```python
from build123d import *

# Parameters (mm, degrees)
SKETCH1_W           = 54.9656
SKETCH1_H           = 29.972
BOSS_EXTRUDE1_DEPTH = 21.4122
SHELL1_T            = -2.2352
SKETCH2_R           = 1.143
CUT_EXTRUDE1_DEPTH  = 38.925806526
SKETCH3_W           = 2.2352
SKETCH3_H           = 25.5016
CUT_EXTRUDE2_DEPTH  = 15.24
SKETCH4_W           = 8.981533828
SKETCH4_H           = 2.2352
SKETCH4_W_2         = 18.352338923
CUT_EXTRUDE3_DEPTH  = 19.177
SKETCH6_W           = 0.635
SKETCH6_H           = 1.8288
BOSS_EXTRUDE2_DEPTH = 5.08


with BuildPart() as part:
    # Sketch1 → Boss-Extrude1 (new body)
    with BuildSketch(Plane.XY):
        Rectangle(SKETCH1_W, SKETCH1_H)
    extrude(amount=BOSS_EXTRUDE1_DEPTH)

    # Shell1
    shell1_openings = [part.faces().sort_by_distance(p)[0] for p in [
        (0, 0, 21.4122),
    ]]
    offset(amount=SHELL1_T, openings=shell1_openings, kind=Kind.INTERSECTION)

    # Sketch2 → Cut-Extrude1 (cut, through all)
    with BuildSketch(Plane(origin=(0, 0, 0), x_dir=(-1, 0, 0), z_dir=(0, 0, -1))):
        with Locations((1.7018, 11.176)):
            Circle(SKETCH2_R)
        with Locations((-11.7856, -11.176)):
            Circle(SKETCH2_R)
        with Locations((15.1892, -11.176)):
            Circle(SKETCH2_R)
    extrude(amount=-CUT_EXTRUDE1_DEPTH, mode=Mode.SUBTRACT)

    # Sketch3 → Cut-Extrude2 (cut)
    with BuildSketch(Plane.XY.offset(21.4122)):
        with Locations((26.3652, 0)):
            Rectangle(SKETCH3_W, SKETCH3_H)
    extrude(amount=-CUT_EXTRUDE2_DEPTH, mode=Mode.SUBTRACT)

    # Sketch4 → Cut-Extrude3 (cut)
    with BuildSketch(Plane.XY.offset(21.4122)):
        with Locations((10.870255505, -13.8684)):
            Rectangle(SKETCH4_W, SKETCH4_H)
        with Locations((4.107846369, 13.8684)):
            Rectangle(SKETCH4_W_2, SKETCH4_H)
    extrude(amount=-CUT_EXTRUDE3_DEPTH, mode=Mode.SUBTRACT)

    # Sketch6 → Boss-Extrude2 (add)
    with BuildSketch(Plane.ZY.offset(27.4828)):
        with Locations((0.3175, 6.4516)):
            Rectangle(SKETCH6_W, SKETCH6_H)
        with Locations((0.3175, -6.2992)):
            Rectangle(SKETCH6_W, SKETCH6_H)
    extrude(amount=BOSS_EXTRUDE2_DEPTH)


solid = part.part
```
Check sheet for the modelled part. Datum: model origin and axes. Units: mm. A direction names the side the tool comes from. Coordinates: 2 decimals unless noted, no trailing zeros. Order: outer loops, then holes, each group sorted by start corner. A loop starts at its lowest first (then second) coordinate and runs counter-clockwise, first axis right, second up. Notation, with made-up numbers: (-11, 3) -> (2, 3) arc R24 ccw to (2, 21) -> close; hole circle Ø8 at (0.25, 75.25). An arc over 180 degrees is marked (long way). Write each question's results on one line, items separated by ' | '. Start each with the question number.
1) Section check C-C (x = -21). Enter the section's corners in (y, z).
2) Material ranges on line 1 along X through (y, z) = (11, 4); line 2 along Y through (x, z) = (18, 4.5); line 3 along X through (y, z) = (-13.5, 10), recorded low to high.
3) Section check D-D (y = 2.25). Enter the section's corners in (x, z).
4) Depth check by flat-ended pin: pin 1 (2.5 mm diameter, centred on y = -13.5, z = 8, fed in from -X); pin 2 (0.5 mm diameter, centred on x = -29.5, z = 0.5, fed in from +Y); pin 3 (0.9 mm diameter, centred on x = -29.5, y = -6.5, fed in from +Z) (3 decimals). Enter the tip coordinate at first touch or a pass-through.
5) Set-up check for faces 4 (the face through (26, 0, 6.172)), 5 (the face through (-25.248, 0, 12)), 6 (the face through (-5.068, 14, 12)): record each of +Z, -Z, +X, -X, +Y, -Y from which the full face is reachable in a straight line by a thin tool's end or side.
6) Section check B-B (x = -29). Enter the section's corners in (y, z) (3 decimals), and give its area (3 significant figures).
7) Section check A-A (z = 14.25). Enter the section's corners in (x, y), and give its area (3 significant figures).
8) Draft check along Y on faces 1 (the face through (0, -14.986, 11)), 2 (the face through (-1.45, 10.06, 1.1)), 3 (the face through (13.284, 14, 12)). Enter one of: pulls with the +Y half, pulls with the -Y half, needs draft (parallel to the pull), parting line crosses it, or undercut.
Checked values:
1) outline: (-14.99, 0) -> (14.99, 0) -> (14.99, 21.41) -> (12.75, 21.41) -> (12.75, 2.24) -> (-12.75, 2.24) -> (-12.75, 21.41) -> (-14.99, 21.41) -> close
2) line 1: -27.48 to -25.25, 25.25 to 27.48 | line 2: -14.99 to -12.75, 12.75 to 14.99 | line 3: -27.48 to 6.38, 15.36 to 27.48
3) outline: (-27.48, 0) -> (27.48, 0) -> (27.48, 6.17) -> (25.25, 6.17) -> (25.25, 2.24) -> (-25.25, 2.24) -> (-25.25, 21.41) -> (-27.48, 21.41) -> close
4) pin 1: x = -27.48 | pin 2: y = 7.37 | pin 3: z = 0.635
5) face 4: +Z, +X | face 5: +Z | face 6: +Z, +Y
6) outline: (-7.214, 0) -> (-5.385, 0) -> (-5.385, 0.635) -> (-7.214, 0.635) -> close; (5.537, 0) -> (7.366, 0) -> (7.366, 0.635) -> (5.537, 0.635) -> close | area: 2.32 mm²
7) outline: (-27.48, -14.99) -> (6.38, -14.99) -> (6.38, -12.75) -> (-25.25, -12.75) -> (-25.25, 12.75) -> (-5.07, 12.75) -> (-5.07, 14.99) -> (-27.48, 14.99) -> close; (13.28, 12.75) -> (27.48, 12.75) -> (27.48, 14.99) -> (13.28, 14.99) -> close; (15.36, -14.99) -> (27.48, -14.99) -> (27.48, -12.75) -> (15.36, -12.75) -> close | area: 242 mm²
8) face 1: pulls with the -Y half | face 2: undercut | face 3: needs draft
